Geometry: final body of the model. Coordinates: model frame, mm. A direction names the side the tool comes from. Give positions to 0.01 mm unless a question says otherwise; leave off trailing zeros. Write each loop counter-clockwise with the first axis right and the second up, starting at its lowest first coordinate (ties: lowest second). Pieces come first, ordered by that corner, then holes. Notation, with made-up numbers: M 87.25,21 L 97.25,21 A21 ccw 97.25,58 Z; hole C -32,-39 d8. An arc over 180 degrees is marked long. Use a Markdown table: item, result. Add a question column.
(1) Reachability of faces 1 (the flat face through (28, 25.5, -38)), 2 (the flat face through (0, 13, -8)), 3 (the cylindrical face through (40.213, 14.436, -37.865)), 4 (the flat face through (28, 15, -35.4)), 5 (the flat face through (3, 15, -3.2)) from +Z, -Z, +X, -X, +Y, -Y: full face, straight path, thin tool, end or side. Return the list, or none.
(2) Cut plane A-A (y = 20.25). Output: boundary loops of the cut face in (x, z) (3 decimals), plus the area to 4 significant figures.
(3) Cut plane C-C (y = 15.25). Output: boundary loops of the cut face in (x, z) (3 decimals), plus the area to 3 significant figures.
(4) Material intervals for L1, parallel to Y at x = 51.75, z = -10.4 (3 decimals); L2, parallel to Z at x = 2, y = 13; L3, parallel to X at y = 10.25, z = -9.7 (3 decimals), sorted ascending.
(5) Cut plane D-D (y = 10.25). Output: boundary loops of the cut face in (x, z) (3 decimals).
(6) Pin query (flat end, axial travel): pin 1 Ø8 at (x, z) = (56.5, -21) entering from +Y; pin 2 Ø5 at (y, z) = (14.5, -28.5) entering from +X; pin 3 Ø3 at (y, z) = (16, -6.5) entering from -X. Return the tip coordinate at first contact, or that it passes through.
(7) Draft query along Z for faces 6 (the flat face through (4, 15, -13.2)), 7 (the flat face through (60.5, 3.5, -13.8)), 8 (the flat face through (52, 15, -3.2)). Return one class per face: released by +Z, released by -Z, zero draft, split by the parting line, or undercut.
(8) Cut plane B-B (x = 38.25). Output: boundary loops of the cut face in (y, z) (3 decimals), plus the area to 3 significant figures.
```python
from build123d import *

# Parameters (mm, degrees)
SKETCH1_W           = 55.5
SKETCH1_H           = 40.4
BASE_DEPTH          = 5
SKETCH2_W           = 55.5
SKETCH2_H           = 25.5
WALL_DEPTH          = 5
SKETCH3_W           = 7
SKETCH3_H           = 20.5
MOUNTINGTABS_DEPTH  = 5
LIPS_REACH          = 75.23
SKETCH5_R           = 2.125
MOUNTINGHOLES_DEPTH = 5
FILLETS_R           = 3.5
SKETCH6_R           = 2.125
THROUGHHOLE_DEPTH   = 5
SKETCH7_R           = 2.125
BOSS_EXTRUDE1_DEPTH = 5
BOSS_EXTRUDE2_START = 12
BOSS_EXTRUDE2_DEPTH = 12


with BuildPart() as part:
    # Sketch1 → base (new body)
    with BuildSketch(Plane(origin=(0, 0, 0), x_dir=(1, 0, 0), z_dir=(0, 1, 0))):
        with Locations((27.75, 20.2)):
            Rectangle(SKETCH1_W, SKETCH1_H)
    extrude(amount=BASE_DEPTH)

    # Sketch2 → wall (add)
    with BuildSketch(Plane(origin=(0, 0, -40.4), x_dir=(-1, 0, 0), z_dir=(0, 0, -1))):
        with Locations((-27.75, 12.75)):
            Rectangle(SKETCH2_W, SKETCH2_H)
    extrude(amount=-WALL_DEPTH)

    # Sketch3 → mountingTabs (add)
    with BuildSketch(Plane.XY.offset(-8.2)):
        with Locations((3.5, 15.25)):
            Rectangle(SKETCH3_W, SKETCH3_H)
        with Locations((52, 15.25)):
            Rectangle(SKETCH3_W, SKETCH3_H)
    extrude(amount=MOUNTINGTABS_DEPTH)

    # lips: up to this face of the body (flat: up to its plane)
    lips_end = Plane(part.part.faces().sort_by_distance((27.75, 12.75, -40.4))[0])
    # Sketch4 → lips (add, up to the picked face)
    with BuildSketch(Plane.XY, mode=Mode.PRIVATE) as lips_sk1:
        with BuildLine():
            Line((0, 0), (-10.208884478, 7.148337868))
            ThreePointArc((-10.208884478, 7.148337868), (-11.894564223, 9.792816133), (-11.218174515, 12.85505036))
            Line((-11.218174515, 12.85505036), (0, 5))
            Line((0, 5), (0, 0))
        make_face()
    lips_tool1 = split(extrude(lips_sk1.sketch, amount=-LIPS_REACH, mode=Mode.PRIVATE), bisect_by=lips_end, keep=Keep.BOTH, mode=Mode.PRIVATE)
    # Sketch4 → lips (add, up to the picked face)
    with BuildSketch(Plane.XY, mode=Mode.PRIVATE) as lips_sk2:
        with BuildLine():
            Line((55.5, 5), (66.718174515, 12.85505036))
            ThreePointArc((66.718174515, 12.85505036), (67.394564223, 9.792816133), (65.708884478, 7.148337868))
            Line((65.708884478, 7.148337868), (55.5, 0))
            Line((55.5, 0), (55.5, 5))
        make_face()
    lips_tool2 = split(extrude(lips_sk2.sketch, amount=-LIPS_REACH, mode=Mode.PRIVATE), bisect_by=lips_end, keep=Keep.BOTH, mode=Mode.PRIVATE)
    add(lips_tool1.solids().sort_by(Axis((-5.839287, 6.590277, 0), (0, 0, -1)))[0])
    add(lips_tool2.solids().sort_by(Axis((61.339287, 6.590277, 0), (0, 0, -1)))[0])

    # Sketch5 → mountingHoles (cut)
    with BuildSketch(Plane.XY.offset(-3.2)):
        with Locations((3.75, 20.25)):
            Circle(SKETCH5_R)
        with Locations(Location((3.75, 10.25, 0), (0, 0, 180))):
            Circle(SKETCH5_R)
        with Locations((51.75, 10.25)):
            Circle(SKETCH5_R)
        with Locations(Location((51.75, 20.25, 0), (0, 0, 180))):
            Circle(SKETCH5_R)
    extrude(amount=-MOUNTINGHOLES_DEPTH, mode=Mode.SUBTRACT)

    # fillets
    fillets_edges = [part.edges().sort_by_distance(p)[0] for p in [
        (0, 25.5, -37.9),
        (55.5, 25.5, -37.9),
        (0, 25.5, -5.7),
        (55.5, 25.5, -5.7),
    ]]
    fillet(fillets_edges, radius=FILLETS_R)

    # Sketch6 → throughHole (cut)
    with BuildSketch(Plane.XY.offset(-35.4)):
        with Locations((38.25, 15.25)):
            Circle(SKETCH6_R)
    extrude(amount=-THROUGHHOLE_DEPTH, mode=Mode.SUBTRACT)

    # Sketch7 → Boss-Extrude1 (add)
    # profile 1 of 2: a face of its own
    with BuildSketch(Plane(origin=(0, 0, -8.2), x_dir=(-1, 0, 0), z_dir=(0, 0, -1))):
        with BuildLine():
            Line((-48.5, 25.5), (-52, 25.5))
            ThreePointArc((-52, 25.5), (-54.474873734, 24.474873734), (-55.5, 22))
            Line((-55.5, 22), (-55.5, 5))
            Line((-55.5, 5), (-48.5, 5))
            Line((-48.5, 5), (-48.5, 25.5))
        make_face()
        with Locations((-51.75, 20.25)):
            Circle(SKETCH7_R, mode=Mode.SUBTRACT)
        with Locations(Location((-51.75, 10.25, 0), (0, 0, 180))):
            Circle(SKETCH7_R, mode=Mode.SUBTRACT)
    # profile 2 of 2: a face of its own
    with BuildSketch(Plane(origin=(0, 0, -8.2), x_dir=(-1, 0, 0), z_dir=(0, 0, -1))):
        with BuildLine():
            Line((0, 5), (0, 22))
            ThreePointArc((0, 22), (-1.025126266, 24.474873734), (-3.5, 25.5))
            Line((-3.5, 25.5), (-7, 25.5))
            Line((-7, 25.5), (-7, 5))
            Line((-7, 5), (0, 5))
        make_face()
        with Locations((-3.75, 10.25)):
            Circle(SKETCH7_R, mode=Mode.SUBTRACT)
        with Locations(Location((-3.75, 20.25, 0), (0, 0, 180))):
            Circle(SKETCH7_R, mode=Mode.SUBTRACT)
    extrude(amount=BOSS_EXTRUDE1_DEPTH)

    # Sketch8 → Boss-Extrude2 (add)
    with BuildSketch(Plane.XY.offset(BOSS_EXTRUDE2_START)):
        with BuildLine():
            Line((0, 0), (55.5, 0))
            Line((55.5, 0), (65.708884478, 7.148337868))
            ThreePointArc((65.708884478, 7.148337868), (67.394564223, 9.792816133), (66.718174515, 12.85505036))
            Line((66.718174515, 12.85505036), (55.5, 5))
            Line((55.5, 5), (0, 5))
            Line((0, 5), (-11.218174515, 12.85505036))
            ThreePointArc((-11.218174515, 12.85505036), (-11.894564223, 9.792816133), (-10.208884478, 7.148337868))
            Line((-10.208884478, 7.148337868), (0, 0))
        make_face()
    extrude(amount=-BOSS_EXTRUDE2_DEPTH)


solid = part.part
```
Answer list:
| question | item | result |
|---|---|---|
| 1 | face 1 | +Z, -Z, +X, -X, +Y |
| 1 | face 2 | +Z, -Z, +Y |
| 1 | face 3 | +Z, -Z |
| 1 | face 4 | +Y |
| 1 | face 5 | +Z, +Y |
| 2 | outline | M 0,-40.4 L 55.5,-40.4 L 55.5,-35.4 L 0,-35.4 Z; M 0,-13.2 L 1.625,-13.2 L 1.625,-3.2 L 0,-3.2 Z; M 5.875,-13.2 L 7,-13.2 L 7,-3.2 L 5.875,-3.2 Z; M 48.5,-13.2 L 49.625,-13.2 L 49.625,-3.2 L 48.5,-3.2 Z; M 53.875,-13.2 L 55.5,-13.2 L 55.5,-3.2 L 53.875,-3.2 Z |
| 2 | area | 332.5 mm² |
| 3 | outline | M 0,-40.4 L 36.125,-40.4 L 36.125,-35.4 L 0,-35.4 Z; M 0,-13.2 L 7,-13.2 L 7,-3.2 L 0,-3.2 Z; M 40.375,-40.4 L 55.5,-40.4 L 55.5,-35.4 L 40.375,-35.4 Z; M 48.5,-13.2 L 55.5,-13.2 L 55.5,-3.2 L 48.5,-3.2 Z |
| 3 | area | 396 mm² |
| 4 | L1 | 0 to 8.125, 12.375 to 18.125, 22.375 to 25.5 |
| 4 | L2 | -40.4 to -35.4, -13.2 to -3.2 |
| 4 | L3 | -11.949 to -7.498, 0 to 1.625, 5.875 to 7, 48.5 to 49.625, 53.875 to 55.5, 62.998 to 67.449 |
| 5 | outline | M -11.949,-40.4 L -7.498,-40.4 L -7.498,12 L -11.949,12 Z; M 0,-40.4 L 55.5,-40.4 L 55.5,-35.4 L 0,-35.4 Z; M 0,-13.2 L 1.625,-13.2 L 1.625,-3.2 L 0,-3.2 Z; M 5.875,-13.2 L 7,-13.2 L 7,-3.2 L 5.875,-3.2 Z; M 48.5,-13.2 L 49.625,-13.2 L 49.625,-3.2 L 48.5,-3.2 Z; M 53.875,-13.2 L 55.5,-13.2 L 55.5,-3.2 L 53.875,-3.2 Z; M 62.998,-40.4 L 67.449,-40.4 L 67.449,12 L 62.998,12 Z |
| 6 | pin 1 | y = 8.5 |
| 6 | pin 2 | x = 67.18 |
| 6 | pin 3 | x = 0 |
| 7 | face 6 | undercut |
| 7 | face 7 | zero draft |
| 7 | face 8 | released by +Z |
| 8 | outline | M 0,-40.4 L 13.125,-40.4 L 13.125,-35.4 L 5,-35.4 L 5,12 L 0,12 Z; M 17.375,-40.4 L 25.5,-40.4 L 25.5,-35.4 L 17.375,-35.4 Z |
| 8 | area | 343 mm² |
